Build history of the part. All positions in model axes, mm. Face numbers are marked on the shaded views. A direction names the side the tool comes from. Round coordinates to 2 decimals unless told otherwise and drop trailing zeros. Write each loop counter-clockwise with the first axis right and the second up, starting at its lowest first coordinate (ties: lowest second). Pieces come first, ordered by that corner, then holes. Notation, with made-up numbers: (4, -11) -> (63, -11) arc R14 cw to (63, 6) -> close; hole circle Ø7 at (34, 45.25). An arc over 180 degrees is marked (long way). Return JSON: item names as keys, results as strings.
from build123d import *

# Parameters (mm, degrees)
SKETCH1_W           = 360
SKETCH1_H           = 300
BOSS_EXTRUDE1_DEPTH = 200
SKETCH2_W           = 350
SKETCH2_H           = 290
CUT_EXTRUDE1_DEPTH  = 195
SKETCH3_W           = 30
SKETCH3_H           = 290
CUT_EXTRUDE2_DEPTH  = 309.058436015
SKETCH4_R           = 7.5
CUT_EXTRUDE3_DEPTH  = 439.292140016
SKETCH5_R           = 2.5
CUT_EXTRUDE4_DEPTH  = 5


with BuildPart() as part:
    # Sketch1 → Boss-Extrude1 (new body)
    with BuildSketch(Plane(origin=(0, 0, 0), x_dir=(1, 0, 0), z_dir=(0, 1, 0))):
        Rectangle(SKETCH1_W, SKETCH1_H)
    extrude(amount=-BOSS_EXTRUDE1_DEPTH)

    # Sketch2 → Cut-Extrude1 (cut)
    with BuildSketch(Plane.XZ.offset(200)):
        Rectangle(SKETCH2_W, SKETCH2_H)
    extrude(amount=-CUT_EXTRUDE1_DEPTH, mode=Mode.SUBTRACT)

    # Sketch3 → Cut-Extrude2 (cut, through all)
    with BuildSketch(Plane(origin=(0, 0, 0), x_dir=(1, 0, 0), z_dir=(0, 1, 0))):
        Rectangle(SKETCH3_W, SKETCH3_H)
    extrude(amount=-CUT_EXTRUDE2_DEPTH, mode=Mode.SUBTRACT)

    # Sketch4 → Cut-Extrude3 (cut, through all)
    with BuildSketch(Plane.ZY.offset(180)):
        with Locations((0, -150)):
            Circle(SKETCH4_R)
    extrude(amount=-CUT_EXTRUDE3_DEPTH, mode=Mode.SUBTRACT)

    # Sketch5 → Cut-Extrude4 (cut)
    with BuildSketch(Plane(origin=(0, 0, 0), x_dir=(1, 0, 0), z_dir=(0, 1, 0))):
        with Locations(Location((-25, 85, 0), (0, 0, 270))):
            Circle(SKETCH5_R)
        with Locations(Location((25, 85, 0), (0, 0, 270))):
            Circle(SKETCH5_R)
        with Locations(Location((25, -85, 0), (0, 0, 270))):
            Circle(SKETCH5_R)
        with Locations(Location((-25, -85, 0), (0, 0, 270))):
            Circle(SKETCH5_R)
    extrude(amount=-CUT_EXTRUDE4_DEPTH, mode=Mode.SUBTRACT)


solid = part.part
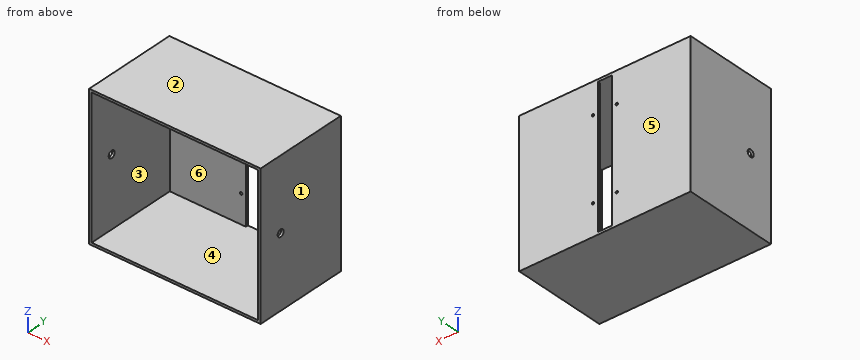
Q1. Wall check: L1, parallel to X at y = -1, z = -85; L2, parallel to X at y = -76.5, z = 9; L3, parallel to Z at x = -148, y = -185.5. Give the ranges that are in metal, low to high.
Verdict:
{"L1": "x = -180 to -27.5, -22.5 to -15, 15 to 22.5, 27.5 to 180", "L2": "x = -180 to -175, 175 to 180", "L3": "z = -150 to -145, 145 to 150"}
Q2. Saw through at A-A on z = -52. List the corners of the cut face in (x, y).
Verdict:
{"outline": "(-180, -200) -> (-175, -200) -> (-175, -5) -> (-15, -5) -> (-15, 0) -> (-180, 0) -> close; (15, -5) -> (175, -5) -> (175, -200) -> (180, -200) -> (180, 0) -> (15, 0) -> close"}
Q3. 3-axis set-ups, long thin cutter, end or side, ignore diameter. For the marked faces 5 and 6: which of +Z, -Z, +X, -X, +Y, -Y reach the whole face in a straight line?
Verdict:
{"face 5": "+Z, -Z, +X, -X, +Y", "face 6": "-Y"}
Q4. Pin check, flat tip, straight feed: pin 1 Ø2 at (x, z) = (40, 91) entering from -Y. Stop position of the tip, or through.
Verdict:
{"pin 1": "stops at y = -5"}
Q5. Saw through at B-B on y = -150. List the corners of the cut face in (x, z).
Verdict:
{"outline": "(-180, -150) -> (180, -150) -> (180, -7.5) -> (175, -7.5) -> (175, -145) -> (-175, -145) -> (-175, -7.5) -> (-180, -7.5) -> close; (-180, 7.5) -> (-175, 7.5) -> (-175, 145) -> (175, 145) -> (175, 7.5) -> (180, 7.5) -> (180, 150) -> (-180, 150) -> close"}
Q6. Saw through at D-D on y = -74.5. List the corners of the cut face in (x, z), then the cut area to 3 significant figures.
Verdict:
{"outline": "(-180, -150) -> (180, -150) -> (180, 150) -> (-180, 150) -> close; hole (-175, -145) -> (175, -145) -> (175, 145) -> (-175, 145) -> close", "area": "6,500 mm²"}
Q7. Two-plate mould, pull along X, no slides. Class the marked faces 1, 2, 3 and 4: +X half, -X half, draft (parallel to the pull), parting line (faces both ways), or undercut.
Verdict:
{"face 1": "+X half", "face 2": "draft", "face 3": "undercut", "face 4": "undercut"}
Q8. Saw through at C-C on z = 0. List the corners of the cut face in (x, y).
Verdict:
{"outline": "(-180, -200) -> (-175, -200) -> (-175, -157.5) -> (-180, -157.5) -> close; (-180, -142.5) -> (-175, -142.5) -> (-175, -5) -> (-15, -5) -> (-15, 0) -> (-180, 0) -> close; (15, -5) -> (175, -5) -> (175, -142.5) -> (180, -142.5) -> (180, 0) -> (15, 0) -> close; (175, -200) -> (180, -200) -> (180, -157.5) -> (175, -157.5) -> close"}
